Check sheet for the modelled part. Datum: model origin and axes. Units: mm. Face numbers are marked on the shaded views. A direction names the side the tool comes from. Round coordinates to 2 decimals unless told otherwise and drop trailing zeros. Order: outer loops, then holes, each group sorted by start corner. A loop starts at its lowest first (then second) coordinate and runs counter-clockwise, first axis right, second up. Notation, with made-up numbers: (16, -26.75) -> (49, -26.75) arc R10 ccw to (49, -8.75) -> close; hole circle Ø2 at (29, 60.25). An arc over 180 degrees is marked (long way). Answer in a Markdown table with one row per item. Add a question column.
1. Sectioned sample at A-A, the plane x = -13. Record the boundary of the cut face in (y, z).
2. Depth check by flat-ended pin: P1, Ø12, axis at x = -8.5, z = 11.5, coming from the +Y side; P2, Ø3.5, axis at y = -0.5, z = 20.5, coming from the -X side; P3, Ø6, axis at x = 6.5, y = -8.5, coming from the +Z side. Enter the tip coordinate at first touch or a pass-through.
3. Access from +Z, -Z, +X, -X, +Y, -Y to the whole of each face (thin tool, end or side, straight path). Record for the marked faces 4, 5, 6, 7 and 8.
4. Draft check along Y on the marked faces 1, 2 and 3. Enter one of: +Y half, -Y half, draft (parallel to the pull), parting line (faces both ways), or undercut.
5. Sectioned sample at B-B, the plane z = 7.5. Count the separate pieces of the cut face and the enclosed holes in it, then the cut area to 3 significant figures.
6. Sectioned sample at C-C, the plane z = 18.5. Record the boundary of the cut face in (x, y).
7. Material ranges on L1, parallel to Y at x = -7, z = 8.5; L2, parallel to Z at x = -13, y = -9.2; L3, parallel to Y at x = 11.5, z = 3, recorded low to high. Write a range as from..to.
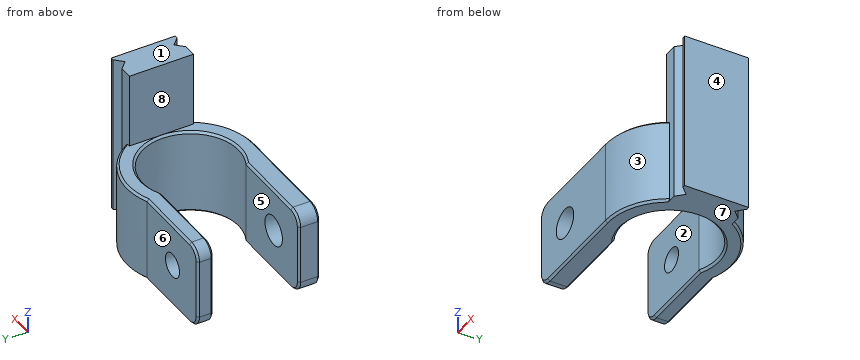
```python
from build123d import *

# Parameters (mm, degrees)
PAD003_DEPTH        = 16
FILLET_R            = 2.5
HOLE002_D           = 4.5
HOLE002_CBORE_D     = 5.6
HOLE002_CBORE_DEPTH = 4.4
CHAMFER005_SIZE     = 0.4
PAD014_DEPTH        = 14


with BuildPart() as part:
    # Sketch015 → Pad003 (new body)
    with BuildSketch(Plane.XY):
        with BuildLine():
            Line((10.392305, 6), (11.8, 6))
            Line((11.8, 6), (13.214214, 4.585786))
            Line((13.214214, 4.585786), (14.628427, 6))
            Line((14.628427, 6), (15.214214, 6))
            Line((15.214214, 6), (15.214214, -6))
            Line((15.214214, -6), (14.628427, -6))
            Line((14.628427, -6), (13.214214, -4.585786))
            Line((13.214214, -4.585786), (11.8, -6))
            Line((11.8, -6), (10.392305, -6))
            ThreePointArc((0, -12), (6, -10.392305), (10.392305, -6))
            Line((0, -12), (-21, -12))
            Line((-21, -12), (-21, -8))
            Line((-21, -8), (-4.123106, -8))
            ThreePointArc((-4.123106, -8), (9, 0), (-4.123106, 8))
            Line((-21, 8), (-4.123106, 8))
            Line((-21, 11), (-21, 8))
            Line((-4.795832, 11), (-21, 11))
            ThreePointArc((10.392305, 6), (3.75235, 11.39824), (-4.795832, 11))
        make_face()
    extrude(amount=PAD003_DEPTH)

    # Fillet
    fillet_edges = [part.edges().sort_by_distance(p)[0] for p in [
        (-21, 9.5, 16),
        (-21, -10, 16),
        (-21, -10, 0),
        (-21, 9.5, 0),
    ]]
    fillet(fillet_edges, radius=FILLET_R)

    # Hole002 (through all)
    with Locations(Plane.XZ.offset(12)):
        with Locations((-13, 8)):
            CounterBoreHole(HOLE002_D / 2, HOLE002_CBORE_D / 2, HOLE002_CBORE_DEPTH)

    # Chamfer005
    chamfer005_edges = [part.edges().sort_by_distance(p)[0] for p in [
        (9, 0, 0),
        (9, 0, 16),
        (-11.311553, 8, 0),
        (-11.311553, -8, 0),
        (3.75235, 11.39824, 0),
        (-11.647916, 11, 0),
        (6, -10.392305, 0),
        (-9.25, -12, 0),
        (3.75235, 11.39824, 16),
        (6, -10.392305, 16),
    ]]
    chamfer(chamfer005_edges, length=CHAMFER005_SIZE)

    # Sketch033 (on Face20 of Pad003) → Pad014 (join)
    with BuildSketch(Plane.XY.offset(16)):
        Polygon((15.214214, 6), (15.214214, -6), (14.628427, -6), (13.214214, -4.585786), (11.8, -6), (9.4, -6), (9.4, 6), (11.8, 6), (13.214214, 4.585786), (14.628427, 6), align=None)
    extrude(amount=PAD014_DEPTH)


solid = part.part
```
Answer key:
| question | item | result |
|---|---|---|
| 1 | outline | (-12, 0.4) -> (-11.6, 0) -> (-8.4, 0) -> (-8, 0.4) -> (-8, 5.2) -> (-12, 5.2) -> close; (-12, 10.8) -> (-8, 10.8) -> (-8, 15.6) -> (-8.4, 16) -> (-11.6, 16) -> (-12, 15.6) -> close; (8, 0.4) -> (8.4, 0) -> (10.6, 0) -> (11, 0.4) -> (11, 5.75) -> (8, 5.75) -> close; (8, 10.25) -> (11, 10.25) -> (11, 15.6) -> (10.6, 16) -> (8.4, 16) -> (8, 15.6) -> close |
| 2 | P1 | stops at y = 11.74 |
| 2 | P2 | stops at x = 9.4 |
| 2 | P3 | stops at z = 16 |
| 3 | face 4 | +Z, -Z, +X, +Y, -Y |
| 3 | face 5 | +Z, -Z, -X |
| 3 | face 6 | +Z, -Z, -X, +Y |
| 3 | face 7 | -Z, +X, -X, +Y, -Y |
| 3 | face 8 | +Z, -X, +Y, -Y |
| 4 | face 1 | draft |
| 4 | face 2 | undercut |
| 4 | face 3 | -Y half |
| 5 | separate pieces | 3 |
| 5 | enclosed holes | 0 |
| 5 | area | 249 mm² |
| 6 | outline | (9.4, -6) -> (11.8, -6) -> (13.21, -4.59) -> (14.63, -6) -> (15.21, -6) -> (15.21, 6) -> (14.63, 6) -> (13.21, 4.59) -> (11.8, 6) -> (9.4, 6) -> close |
| 7 | L1 | y = -12..-8, 8..11 |
| 7 | L2 | z = 0..5.2, 10.8..16 |
| 7 | L3 | y = -6..6 |
